Can you work these out from the model? Positions are in its coordinate system, mm. Face numbers are marked on the shaded views. A direction names the side the tool comes from. Round coordinates to 2 decimals unless told otherwise and drop trailing zeros. Loops run counter-clockwise (first coordinate to the right, second up) from the corner with the lowest first, then second, coordinate; pieces in that order, holes last. Notation, with made-up numbers: M 23,10.5 L 62,10.5 A13 ccw 62,15.5 Z; hole C 71.5,68.5 d11. An arc over 180 degrees is marked long. Use a Markdown table: item, result. Add a question column.
```python
from build123d import *

# Parameters (mm, degrees)
BOSS_EXTRUDE2_DEPTH    = 50
CUT_EXTRUDE1_DEPTH     = 25
SKETCH5_R              = 10
CUT_EXTRUDE3_DEPTH     = 76
SKETCH10_R             = 15
CUT_EXTRUDE4_DEPTH     = 5
CUT_EXTRUDE5_OUTLINE_W = 6.3
CUT_EXTRUDE5_OUTLINE_H = 5.1
CUT_EXTRUDE5_DEPTH     = 10
FILLET1_R              = 0.4
FILLET2_R              = 0.5


# Read off the part's stored shape, not the designer's step: Cut-Extrude5
with BuildPart() as part:
    # Sketch3 → Boss-Extrude2 (new body)
    with BuildSketch(Plane(origin=(0, 0, 0), x_dir=(1, 0, 0), z_dir=(0, 1, 0))):
        with BuildLine():
            Line((5, 44.7), (10.3, 44.7))
            Line((10.3, 44.7), (10.3, 47.2))
            Line((10.3, 47.2), (15, 44.486453735))
            Line((15, 44.486453735), (15, 43.7))
            Line((15, 43.7), (5, 43.7))
            Line((5, 43.7), (5, 6.3))
            Line((5, 6.3), (15, 6.3))
            Line((15, 6.3), (15, 5.513546265))
            Line((15, 5.513546265), (10.3, 2.8))
            Line((10.3, 2.8), (10.3, 5.3))
            Line((10.3, 5.3), (5, 5.3))
            Line((5, 5.3), (5, 0))
            Line((5, 0), (0, 0))
            Line((0, 0), (-25, 0))
            ThreePointArc((-25, 0), (-50, 25), (-25, 50))
            Line((-25, 50), (0, 50))
            Line((0, 50), (5, 50))
            Line((5, 50), (5, 44.7))
        make_face()
    extrude(amount=BOSS_EXTRUDE2_DEPTH)

    # Sketch4 → Cut-Extrude1 (cut)
    with BuildSketch(Plane(origin=(0, 50, 0), x_dir=(1, 0, 0), z_dir=(0, 1, 0))):
        Polygon((0, 0), (-50, 0), (-50, 50), (0, 50), (0.5, 50), (0.5, 0), align=None)
    extrude(amount=-CUT_EXTRUDE1_DEPTH, mode=Mode.SUBTRACT)

    # Sketch5 → Cut-Extrude3 (cut, through all)
    with BuildSketch(Plane(origin=(0, 25, 0), x_dir=(1, 0, 0), z_dir=(0, 1, 0))):
        with Locations(Location((-25, 25, 0), (0, 0, 270))):
            Circle(SKETCH5_R)
    extrude(amount=-CUT_EXTRUDE3_DEPTH, mode=Mode.SUBTRACT)

    # Sketch10 → Cut-Extrude4 (cut)
    with BuildSketch(Plane.XZ):
        with Locations(Location((-25, -25, 0), (0, 0, 270))):
            Circle(SKETCH10_R)
    extrude(amount=-CUT_EXTRUDE4_DEPTH, mode=Mode.SUBTRACT)

    # Cut-Extrude5 outline → Cut-Extrude5 (cut)
    with BuildSketch(Plane(origin=(5, 0, 0), x_dir=(0, 0, -1), z_dir=(1, 0, 0))):
        with Locations((3.15, 47.45)):
            Rectangle(CUT_EXTRUDE5_OUTLINE_W, CUT_EXTRUDE5_OUTLINE_H)
        with Locations((3.15, 2.55)):
            Rectangle(CUT_EXTRUDE5_OUTLINE_W, CUT_EXTRUDE5_OUTLINE_H)
        with Locations((46.85, 47.45)):
            Rectangle(CUT_EXTRUDE5_OUTLINE_W, CUT_EXTRUDE5_OUTLINE_H)
        with Locations((46.85, 2.55)):
            Rectangle(CUT_EXTRUDE5_OUTLINE_W, CUT_EXTRUDE5_OUTLINE_H)
    extrude(amount=CUT_EXTRUDE5_DEPTH, mode=Mode.SUBTRACT)

    # Fillet1
    fillet1_edges = [part.edges().sort_by_distance(p)[0] for p in [
        (15, 25, -44.486453735),
        (15, 25, -43.7),
        (15, 25, -6.3),
        (15, 25, -5.513546265),
    ]]
    fillet(fillet1_edges, radius=FILLET1_R)

    # Fillet2
    fillet2_edges = [part.edges().sort_by_distance(p)[0] for p in [
        (10.3, 25, -47.2),
        (10.3, 25, -2.8),
    ]]
    fillet(fillet2_edges, radius=FILLET2_R)


solid = part.part
```
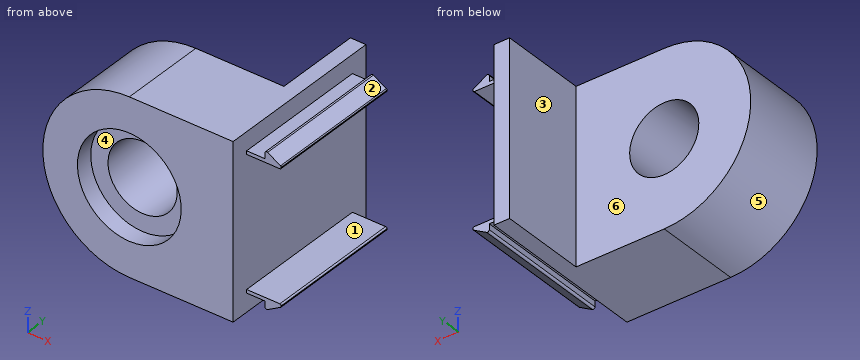
(1) Thinking about a two-plate mould opening in X: for the marked faces 4, 5 and 6, which applies, released by +X, released by -X, zero draft, split by the parting line, or undercut?
(2) Suppose I cut it at C-C on x = -13.5. List the corners of the cut face in (y, z) for me.
(3) Suppose I cut it at A-A on z = -25. List the corners of the cut face in (x, y) for me, and give its area (4 significant figures).
(4) I'm going to push flat-ended pins straight in: pin 1 (1 mm diameter, centred on x = -3, z = -18, fed in from -Y); pin 2 (1.5 mm diameter, centred on x = -16, z = -17, fed in from +Y); pin 3 (4 mm diameter, centred on x = -43, y = 9, fed in from -Z); pin 4 (4 mm diameter, centred on x = 7.5, y = 21, fed in from -Z). Where does each tip first touch, or does it pass through?
(5) Suppose I cut it at B-B on y = 21.5. List the corners of the cut face in (x, z) for me, and give its area (3 significant figures).
(6) If I drill on probe 1 along X at (y, z) = (3.9, -25); probe 2 along X at (y, z) = (12.5, -25); probe 3 along Y at (x, z) = (-13.5, -15.5), over which ranges is the centre line in solid material (lowest first)? Write a range as [from, to].
(7) On a 3-axis mill with a long thin cutter (end or side, diameter ignored), from which of +Z, -Z, +X, -X, +Y, -Y can I reach the whole of each face in a straight line? I mean the marked faces 1, 2 and 3. Say none if no direction works.
(8) Suppose I cut it at D-D on y = 35. List the corners of the cut face in (x, z) for me.
Results below:
| question | item | result |
|---|---|---|
| 1 | face 4 | undercut |
| 1 | face 5 | released by -X |
| 1 | face 6 | zero draft |
| 2 | outline | M 0,-50 L 25,-50 L 25,0 L 0,0 L 0,-15.37 L 5,-15.37 L 5,-34.63 L 0,-34.63 Z |
| 3 | outline | M -50,0 L -40,0 L -40,5 L -35,5 L -35,25 L -50,25 Z; M -15,5 L -10,5 L -10,0 L 5,0 L 5,50 L 0.5,50 L 0.5,25 L -15,25 Z |
| 3 | area | 937.5 mm² |
| 4 | pin 1 | stops at y = 0 |
| 4 | pin 2 | stops at y = 25 |
| 4 | pin 3 | stops at z = -44.21 |
| 4 | pin 4 | stops at z = -44.7 |
| 5 | outline | M -25,-50 L 5,-50 L 5,-44.7 L 10.3,-44.7 L 10.3,-46.33 A0.5 ccw 11.05,-46.77 L 14.8,-44.6 A0.4 ccw 15,-44.26 L 15,-44.1 A0.4 ccw 14.6,-43.7 L 5,-43.7 L 5,-6.3 L 14.6,-6.3 A0.4 ccw 15,-5.9 L 15,-5.74 A0.4 ccw 14.8,-5.4 L 11.05,-3.23 A0.5 ccw 10.3,-3.67 L 10.3,-5.3 L 5,-5.3 L 5,0 L -25,0 A25 ccw Z; hole C -25,-25 d20 |
| 5 | area | 2,200 mm² |
| 6 | probe 1 | x = [-50, -40], [-10, 5] |
| 6 | probe 2 | x = [-50, -35], [-15, 5] |
| 6 | probe 3 | y = [5, 25] |
| 7 | face 1 | +X, +Y, -Y |
| 7 | face 2 | +Z, +X, +Y, -Y |
| 7 | face 3 | +Z, -Z, -X, +Y |
| 8 | outline | M 0.5,-50 L 5,-50 L 5,-44.7 L 10.3,-44.7 L 10.3,-46.33 A0.5 ccw 11.05,-46.77 L 14.8,-44.6 A0.4 ccw 15,-44.26 L 15,-44.1 A0.4 ccw 14.6,-43.7 L 5,-43.7 L 5,-6.3 L 14.6,-6.3 A0.4 ccw 15,-5.9 L 15,-5.74 A0.4 ccw 14.8,-5.4 L 11.05,-3.23 A0.5 ccw 10.3,-3.67 L 10.3,-5.3 L 5,-5.3 L 5,0 L 0.5,0 Z |
